Verification items for the finished model (mm, model axes). Face numbers are marked on the shaded views. A direction names the side the tool comes from. Give positions to 0.01 mm unless a question says otherwise; leave off trailing zeros. Order: outer loops, then holes, each group sorted by start corner. A loop starts at its lowest first (then second) coordinate and runs counter-clockwise, first axis right, second up. Notation, with made-up numbers: (8, 31) -> (13, 31) arc R20 cw to (13, 49) -> close; hole circle Ø7 at (78, 28). An arc over 180 degrees is marked (long way). One line per question, with ' | ' between items. Start each with the question number.
Q1. Mould release check, pull along X, two halves, no side actions. Record for the marked faces 1, 2 and 3: released by +X, released by -X, zero draft, split by the parting line, or undercut.
Q2. Material ranges on probe 1 along X at (y, z) = (-4.25, 5.5); probe 2 along X at (y, z) = (-9.75, 3.75); probe 3 along X at (y, z) = (-7.5, 5), recorded low to high. Write a range as [from, to].
Q3. Section check B-B on z = 2. Record the cut outline in (x, y).
Q4. Access from +Z, -Z, +X, -X, +Y, -Y to the whole of each face (thin tool, end or side, straight path). Record for the marked faces 4, 5 and 6.
Q5. Section check C-C on y = -7.5. Record the cut outline in (x, z), plus the area to 3 significant figures.
Q6. Section check A-A on y = -10. Record the cut outline in (x, z).
Q7. Go/stop test with flat-tipped pins: pin 1 (1 mm diameter, centred on y = -6.5, z = 4, fed in from -X); pin 2 (1.8 mm diameter, centred on x = -10.5, z = 2, fed in from +Y); pin 3 (0.7 mm diameter, centred on x = 3, z = 2, fed in from +Y). Record where each tip stops, or that it passes through.
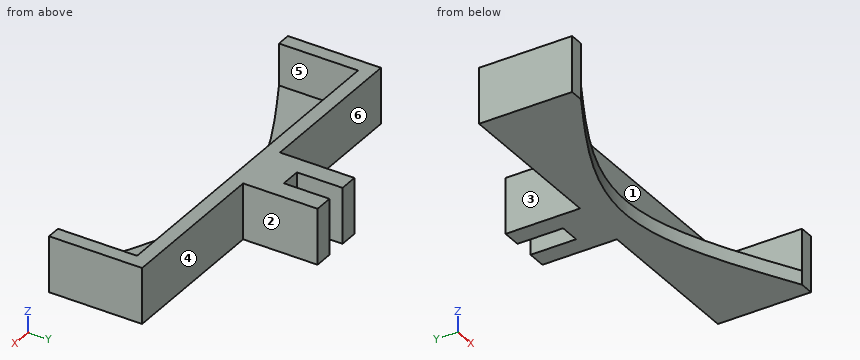
from build123d import *

# Parameters (mm, degrees)
F1_DEPTH = 6
F2_DEPTH = 1.5


with BuildPart() as f1:
    # F0 (on Top) → F1 (new body)
    with BuildSketch(Plane.XY):
        Polygon((2, 0), (0, 0), (0, -8), (-17, -8), (-17, -18), (-15.5, -18), (-15.5, -9.5), (21.7, -9.5), (21.7, -18), (23.2, -18), (23.2, -8), (6.2, -8), (6.2, 0), (4.2, 0), (4.2, -4.9), (2, -4.9), align=None)
    extrude(amount=F1_DEPTH)

    # F0 (on Top) → F2 (join)
    with BuildSketch(Plane.XY):
        with BuildLine():
            Line((-15.5, -9.5), (-15.5, -18))
            add(Edge.make_bspline(
                [(-15.5, -18), (-9.133333, -14.471125), (3.1, -7.413374), (15.333333, -14.471125), (21.7, -18)],
                knots=[0, 0, 0, 0, 19.894015, 39.78803, 39.78803, 39.78803, 39.78803], degree=3))
            Line((21.7, -18), (21.7, -9.5))
            Line((21.7, -9.5), (-15.5, -9.5))
        make_face()
    extrude(amount=F2_DEPTH)


solid = f1.part
Filled in:
1) face 1: undercut | face 2: released by +X | face 3: released by -X
2) probe 1: [0, 2], [4.2, 6.2] | probe 2: [-17, -15.5], [21.7, 23.2] | probe 3: [0, 6.2]
3) outline: (-17, -18) -> (-15.5, -18) -> (-15.5, -9.5) -> (21.7, -9.5) -> (21.7, -18) -> (23.2, -18) -> (23.2, -8) -> (6.2, -8) -> (6.2, 0) -> (4.2, 0) -> (4.2, -4.9) -> (2, -4.9) -> (2, 0) -> (0, 0) -> (0, -8) -> (-17, -8) -> close
4) face 4: +Z, -Z, +X, +Y | face 5: +Z, -Y | face 6: +Z, -Z, -X, +Y
5) outline: (0, 0) -> (6.2, 0) -> (6.2, 6) -> (0, 6) -> close | area: 37.2 mm²
6) outline: (-17, 0) -> (23.2, 0) -> (23.2, 6) -> (21.7, 6) -> (21.7, 1.5) -> (-15.5, 1.5) -> (-15.5, 6) -> (-17, 6) -> close
7) pin 1: x = 0 | pin 2: y = -8 | pin 3: y = -4.9
